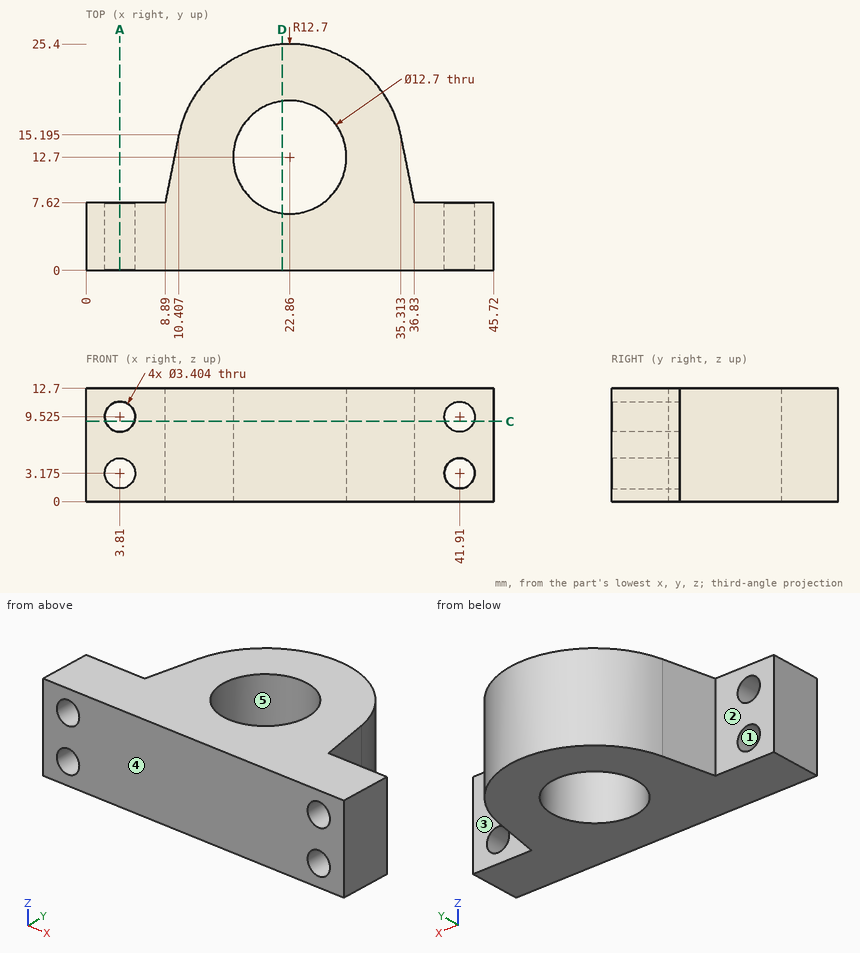
Geometry: see drawing. Coordinates: mm, zero at the bounding-box minimum. A direction names the side the tool comes from. Coordinates: 2 decimals unless noted, no trailing zeros. Loops run counter-clockwise (first coordinate to the right, second up) from the corner with the lowest first, then second, coordinate; pieces in that order, holes last.
Q1. Cut plane A-A (x = 3.81). Output: boundary loops of the cut face in (y, z).
Q2. Material intervals for line 1 (X direction, y = 10.5, z = 2.5); line 2 (X direction, y = 15.25, z = 10.25) (1 decimal); line 3 (Y direction, x = 6, z = 10.75), sorted ascending.
Q3. Cut plane C-C (z = 9). Give the number of separate pieces and of enclosed holes in the cut face, then the cut area to 3 significant figures.
Q4. Set-up query: the marked faces 1 and 2. Return all of +Z, -Z, +X, -X, +Y, -Y with unobstructed straight access to the full face (end or side cutting, diameter ignored); none if empty.
Q5. Cut plane D-D (x = 22). Output: boundary loops of the cut face in (y, z), then the cut area to 3 significant figures.
Q6. Contact query for flat-ended pins moving along their axis: pin 1 (3 mm diameter, centred on x = 5, z = 6.5, fed in from +Y); pin 2 (3 mm diameter, centred on y = 17.5, z = 4, fed in from -X); pin 3 (6 mm diameter, centred on y = 15.5, z = 2, fed in from +X). Output: stop coordinate, or through.
Q7. Draft query along Y for the marked faces 3, 4 and 5. Return one class per face: +Y half, -Y half, draft (parallel to the pull), parting line (faces both ways), or undercut.
Working result:
1. outline: (0, 0) - (7.62, 0) - (7.62, 1.47) - (0, 1.47) - close; (0, 4.88) - (7.62, 4.88) - (7.62, 7.82) - (0, 7.82) - close; (0, 11.23) - (7.62, 11.23) - (7.62, 12.7) - (0, 12.7) - close
2. line 1: x = 9.47 to 16.9, 28.82 to 36.25
2. line 2: x = 10.4 to 17, 28.7 to 35.3
2. line 3: y = 0 to 7.62
3. separate pieces: 3
3. enclosed holes: 1
3. area: 563 mm2
4. face 1: +Y, -Y
4. face 2: +Z, -Z, -X, +Y
5. outline: (0, 0) - (6.41, 0) - (6.41, 12.7) - (0, 12.7) - close; (18.99, 0) - (25.37, 0) - (25.37, 12.7) - (18.99, 12.7) - close
5. area: 162 mm2
6. pin 1: stops at y = 7.62
6. pin 2: stops at x = 10.6
6. pin 3: stops at x = 35.85
7. face 3: +Y half
7. face 4: -Y half
7. face 5: undercut
